```python
from build123d import *

# Parameters (mm, degrees)
BOSS_EXTRUDE1_DEPTH      = 12.7
BOSS_EXTRUDE2_DEPTH      = 6.35
BOSS_EXTRUDE2_DEPTH_BACK = 19.05
SKETCH3_R                = 3.1496
SKETCH4_R                = 3.175
CUT_EXTRUDE1_DEPTH       = 30.854524808


with BuildPart() as part:
    # Sketch1 → Boss-Extrude1 (new body)
    with BuildSketch(Plane.XY):
        with BuildLine():
            Line((0, 0), (0, 12.7))
            ThreePointArc((0, 12.7), (-16.624515829, 6.35), (0, 0))
        make_face()
    extrude(amount=BOSS_EXTRUDE1_DEPTH)

    # Sketch3 → Boss-Extrude2 (add, two sides: drawn at the far end of the back side and taken through both)
    with BuildSketch(Plane.XY.offset(12.7).offset(-BOSS_EXTRUDE2_DEPTH_BACK)):
        with Locations((-7.099515829, 6.35)):
            Circle(SKETCH3_R)
    extrude(amount=BOSS_EXTRUDE2_DEPTH + BOSS_EXTRUDE2_DEPTH_BACK)

    # Sketch4 → Cut-Extrude1 (cut, through all)
    with BuildSketch(Plane(origin=(0, 0, 0), x_dir=(0, 0, -1), z_dir=(1, 0, 0))):
        with Locations((-6.35, 6.35)):
            Circle(SKETCH4_R)
    extrude(amount=-CUT_EXTRUDE1_DEPTH, mode=Mode.SUBTRACT)


solid = part.part
```
Verification items for the finished model (mm, model axes). A direction names the side the tool comes from. Coordinates: 2 decimals unless noted, no trailing zeros. Loops run counter-clockwise (first coordinate to the right, second up) from the corner with the lowest first, then second, coordinate; pieces in that order, holes last. Notation, with made-up numbers: (69.25, 2.5) -> (82.25, 2.5) arc R30 cw to (82.25, 30.5) -> close; hole circle Ø1 at (19.25, -1). An arc over 180 degrees is marked (long way). Answer in a Markdown table with one row per item. Add a question column.
1. Material ranges on probe 1 along Z at (x, y) = (-10.5, 6.35) (3 decimals); probe 2 along Z at (x, y) = (-4.25, 14.5); probe 3 along Y at (x, z) = (-13, 6.35) (3 decimals), recorded low to high. Write a range as [from, to].
2. Section check B-B, the plane x = -12.5. Enter the section's corners in (y, z) (3 decimals).
3. Access from +Z, -Z, +X, -X, +Y, -Y to the whole of each face (thin tool, end or side, straight path). Record for faces 4 (the face through (-7.51, 9.473, 15.831)), 5 (the face through (-7.51, 9.473, -3.219)), 6 (the face through (-7, 6, -6.35)).
4. Section check D-D, the plane z = -2. Enter the section's corners in (x, y), then the cut area to 3 significant figures.
5. Section check C-C, the plane z = 6.35. Enter the section's corners in (x, y) (3 decimals), then the cut area to 3 significant figures.
6. Draft check along Z on faces 1 (the face through (-7, 6, 19.05)), 2 (the face through (-8.2, 9, 4.6)), 3 (the face through (-10, 4, 0)). Enter one of: +Z half, -Z half, draft (parallel to the pull), parting line (faces both ways), or undercut.
7. Depth check by flat-ended pin: P1, Ø4, axis at x = -13, z = 8, coming from the -Y side; P2, Ø1, axis at y = 0, z = 7, coming from the -X side; P3, Ø3, axis at y = 10.5, z = 15.5, coming from the -X side. Enter the tip coordinate at first touch or a pass-through.
8. Section check A-A, the plane y = 6.35. Enter the section's corners in (x, z) (3 decimals).
Derived:
| question | item | result |
|---|---|---|
| 1 | probe 1 | z = [0, 3.175], [9.525, 12.7] |
| 1 | probe 2 | z = [0, 12.7] |
| 1 | probe 3 | y = [-1.127, 3.175], [9.525, 13.827] |
| 2 | outline | (-1.496, 0) -> (14.196, 0) -> (14.196, 12.7) -> (-1.496, 12.7) -> close; hole circle Ø6.35 at (6.35, 6.35) |
| 3 | face 4 | +Z |
| 3 | face 5 | -Z |
| 3 | face 6 | -Z, +X, -X, +Y, -Y |
| 4 | outline | circle Ø6.3 at (-7.1, 6.35) |
| 4 | area | 31.2 mm² |
| 5 | outline | (-16.08, 3.175) arc R9.525 ccw to (0, 0) -> (0, 3.175) -> close; (-16.08, 9.525) -> (0, 9.525) -> (0, 12.7) arc R9.525 ccw to start |
| 5 | area | 159 mm² |
| 6 | face 1 | +Z half |
| 6 | face 2 | undercut |
| 6 | face 3 | -Z half |
| 7 | P1 | stops at y = -2.34 |
| 7 | P2 | stops at x = -14.62 |
| 7 | P3 | stops at x = -8.8 |
| 8 | outline | (-16.625, 0) -> (-10.249, 0) -> (-10.249, -6.35) -> (-3.95, -6.35) -> (-3.95, 0) -> (0, 0) -> (0, 3.175) -> (-16.625, 3.175) -> close; (-16.625, 9.525) -> (0, 9.525) -> (0, 12.7) -> (-3.95, 12.7) -> (-3.95, 19.05) -> (-10.249, 19.05) -> (-10.249, 12.7) -> (-16.625, 12.7) -> close |
